from build123d import *

# Parameters (mm, degrees)
BOSS_EXTRUDE1_DEPTH                             = 4.699
CSK_FOR_M3_FLAT_HEAD_MACHINE_SCREW1_D           = 3.4
CSK_FOR_M3_FLAT_HEAD_MACHINE_SCREW1_CSINK_D     = 6.3
CSK_FOR_M3_FLAT_HEAD_MACHINE_SCREW1_CSINK_ANGLE = 90
BOSS_EXTRUDE2_DEPTH                             = 17.476
FILLET1_R                                       = 3.5


# Read off the part's stored shape, not the designer's step: Mirror1
with BuildPart() as part:
    # Sketch1 → Boss-Extrude1 (new body)
    with BuildSketch(Plane(origin=(0, 0, 0), x_dir=(1, 0, 0), z_dir=(0, 1, 0))):
        with BuildLine():
            ThreePointArc((-29.559395906245367, 40.016304347826086), (-1.9222382209583215, 49.71285045359888), (26.381150789265686, 42.17934782608695))
            ThreePointArc((26.381150789265686, 42.17934782608695), (27.57196966138789, 37.011471046035254), (22.404092881336187, 35.82065217391305))
            ThreePointArc((22.404092881336187, 35.82065217391305), (-1.6324535645324438, 42.21845088772971), (-25.10320556862043, 33.983695652173914))
            ThreePointArc((-25.10320556862043, 33.983695652173914), (-30.347605085258984, 34.771904831187534), (-29.559395906245367, 40.016304347826086))
        make_face()
    extrude(amount=BOSS_EXTRUDE1_DEPTH)

    # CSK for M3 Flat Head Machine Screw1 (through all)
    with Locations(Plane(origin=(0, 4.699, 0), x_dir=(1, 0, 0), z_dir=(0, 1, 0))):
        with Locations((-27.331300737, 37), (24.392621835, 39)):
            CounterSinkHole(CSK_FOR_M3_FLAT_HEAD_MACHINE_SCREW1_D / 2, CSK_FOR_M3_FLAT_HEAD_MACHINE_SCREW1_CSINK_D / 2, counter_sink_angle=CSK_FOR_M3_FLAT_HEAD_MACHINE_SCREW1_CSINK_ANGLE)

    # Sketch4 → Boss-Extrude2 (add)
    with BuildSketch(Plane(origin=(0, 4.699, 0), x_dir=(1, 0, 0), z_dir=(0, 1, 0))):
        with BuildLine():
            Line((-22.05301335725447, 36.037856510408), (-25.967749456175376, 42.43510914539167))
            ThreePointArc((-25.967749456175376, 42.43510914539167), (-1.9222382209583215, 49.71285045359888), (22.613452452482438, 44.31359010709148))
            Line((22.613452452482438, 44.31359010709148), (19.204389268691116, 37.633149387429455))
            ThreePointArc((19.204389268691116, 37.633149387429455), (-1.6324535645324438, 42.21845088772971), (-22.05301335725447, 36.037856510408))
        make_face()
    extrude(amount=BOSS_EXTRUDE2_DEPTH)

    # Mirror1: part across plane


with BuildPart() as part_1:
    add(part.part)
    add(part.part.mirror(Plane(origin=(12.196310917650468, 22.175, -19.5), x_dir=(0, 0, 1), z_dir=(0, -1, 0))))

    # Fillet1
    fillet1_edges = [part_1.edges().sort_by_distance(p)[0] for p in [
        (19.204389268691116, 22.175000000000004, -37.633149387429455),
        (-22.053013357254475, 22.175, -36.037856510408005),
        (-25.967749456175373, 22.175000000000004, -42.43510914539168),
        (22.613452452482434, 22.175, -44.313590107091485),
    ]]
    fillet(fillet1_edges, radius=FILLET1_R)


solid = part_1.part
CAD build for the part. Positions are in the model's coordinates, mm. A direction names the side the tool comes from. Give positions to 0.01 mm unless a question says otherwise; leave off trailing zeros. Order: outer loops, then holes, each group sorted by start corner. A loop starts at its lowest first (then second) coordinate and runs counter-clockwise, first axis right, second up. Notation, with made-up numbers: (21.5, -9) -> (67.5, -9) arc R22 cw to (67.5, 3) -> close; hole circle Ø5 at (-28.75, 10). An arc over 180 degrees is marked (long way). Return JSON: item names as keys, results as strings.
Q1. Which spindle directions (+Z, -Z, +X, -X, +Y, -Y) get a long thin tool onto all of the face, cutting with end or side? Do faces 5 (the face through (18.789, 21.93, -38.924)), 6 (the face through (24.76, 42.75, -37.34)), 7 (the face through (-24.444, 22.42, -42.15)). Say none if no direction does.
Working result:
{"face 5": "+Z", "face 6": "+Y, -Y", "face 7": "-X"}
Q2. Saw through at A-A (x = 17). Write the cut outline in (y, z).
Working result:
{"outline": "(0, -46.76) -> (44.35, -46.76) -> (44.35, -38.68) -> (39.65, -38.68) -> (39.65, -38.78) -> (4.7, -38.78) -> (4.7, -38.68) -> (0, -38.68) -> close"}
Q3. Saw through at B-B (y = 29). Write the cut outline in (x, z).
Working result:
{"outline": "(-24.07, -39.34) arc R3.5 ccw to (-22.68, -44.28) arc R49.75 ccw to (19.2, -45.9) arc R3.5 ccw to (20.96, -41.08) -> (20.73, -40.63) arc R3.5 ccw to (16.27, -38.99) arc R42.25 cw to (-19.23, -37.62) arc R3.5 ccw to (-23.81, -38.91) -> close"}
Q4. Flat gauge pins, fed straight in: pin 1 (2.5 mm diameter, centred on x = 24.39, z = -39, fed in from -Y); pin 2 (1 mm diameter, centred on y = 12, z = -43.5, fed in from +X); pin 3 (5 mm diameter, centred on x = 6, y = 20.5, fed in from +Z); pin 4 (3 mm diameter, centred on y = 8, z = -40, fed in from -X). Where does each tip first touch, or does it go through?
Working result:
{"pin 1": "through", "pin 2": "x = 21.33", "pin 3": "z = -41.39", "pin 4": "x = -24.59"}
Q5. Saw through at C-C (x = 3.5). Write the cut outline in (y, z).
Working result:
{"outline": "(0, -49.63) -> (44.35, -49.63) -> (44.35, -42.1) -> (0, -42.1) -> close"}
Q6. Mould opens along Z. For faces 1 (the face through (27.615, 42.033, -37.082)), 2 (the face through (-24, 39.651, -38)), 3 (the face through (-25.98, 42.75, -35.97)), 4 (the face through (-1.28, 22.49, -42.23)) say: pulls with the +Z half, pulls with the -Z half, needs draft (parallel to the pull), parting line crosses it, or undercut.
Working result:
{"face 1": "parting line crosses it", "face 2": "needs draft", "face 3": "undercut", "face 4": "pulls with the +Z half"}
Q7. Saw through at D-D (x = -14). Write the cut outline in (y, z), then the cut area to 3 significant figures.
Working result:
{"outline": "(0, -47.74) -> (44.35, -47.74) -> (44.35, -39.86) -> (0, -39.86) -> close", "area": "349 mm²"}
Q8. Drill centre lines: line 1 (X direction, y = 2.45, z = -37); line 2 (X direction, y = 0.8, z = -39); line 3 (Z direction, x = -20.5, y = 14). Where is each one in solid material? Low to high.
Working result:
{"line 1": "-31.08 to -29.03, -25.63 to -20.4, 20.4 to 27.56", "line 2": "-30.5 to -16.25, 16.25 to 22.69, 26.09 to 28.14", "line 3": "-45.33 to -37.25"}
